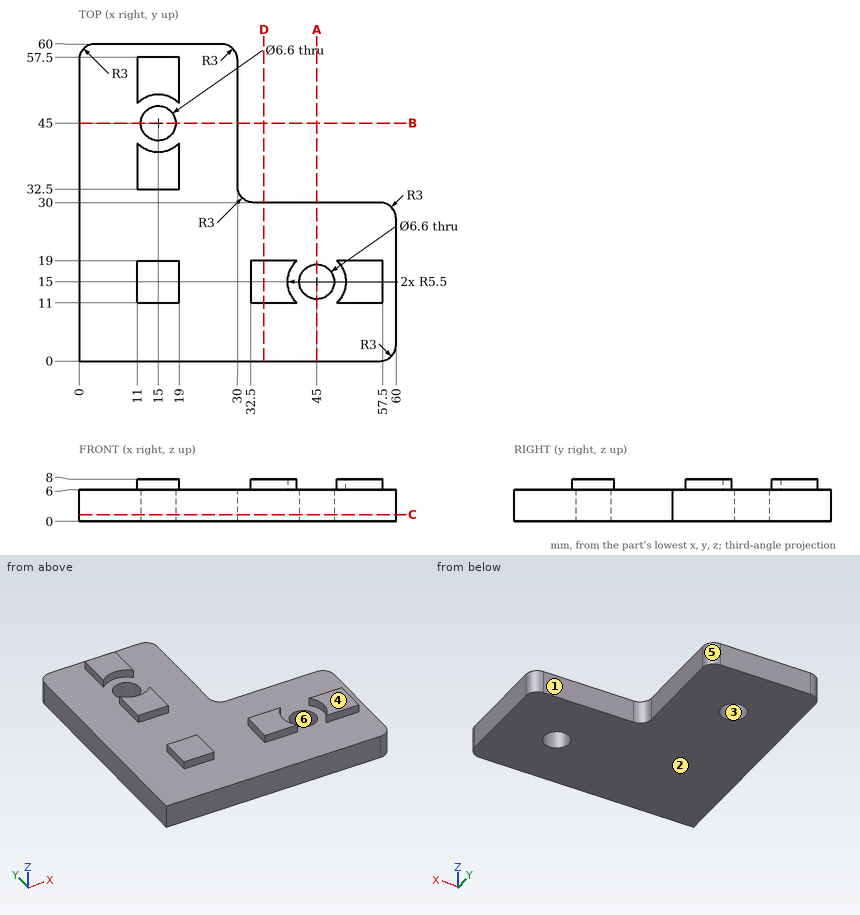
Job drawing, mm, ordinate dimensions from the low corner. One solid piece. A direction names the side the tool comes from. Round coordinates to 2 decimals unless told otherwise and drop trailing zeros. Loops run counter-clockwise (first coordinate to the right, second up) from the corner with the lowest first, then second, coordinate; pieces in that order, holes last. Notation, with made-up numbers: (50.5, 61) -> (107.5, 61) arc R17 ccw to (107.5, 77) -> close; hole circle Ø4 at (88.25, 69). An arc over 180 degrees is marked (long way). Use CSV: the item, a comma, the result in double quotes. Start each with the question number.
Q1. Saw through at A-A on x = 45. Give the cut face in (y, z), and give its area (3 significant figures).
Q2. Drill centre lines: L1, parallel to Y at x = 45, z = 4.75; L2, parallel to Z at x = 19.5, y = 52; L3, parallel to X at y = 14.5, z = 7.5. Where is each one in solid material? Low to high.
Q3. Which spindle directions (+Z, -Z, +X, -X, +Y, -Y) get a long thin tool onto all of the face, cutting with end or side? Do the marked faces 1 and 2. Say none if no direction does.
Q4. Saw through at D-D on x = 35. Give the cut face in (y, z).
Q5. Flat gauge pins, fed straight in: pin 1 Ø0.6 at (y, z) = (16.5, 6.5) entering from -X; pin 2 Ø0.6 at (y, z) = (16.5, 7) entering from +X; pin 3 Ø1 at (x, y) = (41.5, 31) entering from -Z; pin 4 Ø1.6 at (x, z) = (13, 7) entering from -Y. Where does each tip first touch, or does it go through?
Q6. Mould opens along X. For the marked faces 3, 4, 5 and 6 say: +X half, -X half, draft (parallel to the pull), parting line (faces both ways), or undercut.
Q7. Saw through at C-C on z = 1.25. Give the cut face in (x, y).
Solutions:
1,outline,"(0, 0) -> (11.7, 0) -> (11.7, 6) -> (0, 6) -> close; (18.3, 0) -> (30, 0) -> (30, 6) -> (18.3, 6) -> close"
1,area,"140 mm^2"
2,L1,"y = 0 to 11.7, 18.3 to 30"
2,L2,"z = 0 to 6"
2,L3,"x = 11 to 19, 32.5 to 39.52, 50.48 to 57.5"
3,face 1,"+Z, -Z, +X, +Y"
3,face 2,"-Z, +X, -X, +Y, -Y"
4,outline,"(0, 0) -> (30, 0) -> (30, 6) -> (19, 6) -> (19, 8) -> (11, 8) -> (11, 6) -> (0, 6) -> close"
5,pin 1,"stops at x = 11"
5,pin 2,"stops at x = 57.5"
5,pin 3,"passes through"
5,pin 4,"stops at y = 11"
6,face 3,"undercut"
6,face 4,"draft"
6,face 5,"+X half"
6,face 6,"undercut"
7,outline,"(0, 0) -> (57, 0) arc R3 ccw to (60, 3) -> (60, 27) arc R3 ccw to (57, 30) -> (33, 30) arc R3 cw to (30, 33) -> (30, 57) arc R3 ccw to (27, 60) -> (3, 60) arc R3 ccw to (0, 57) -> close; hole circle Ø6.6 at (15, 45); hole circle Ø6.6 at (45, 15)"
